Here's how the part is built. I have some questions about the finished solid (model axes, mm). A direction names the side the tool comes from. Round coordinates to 2 decimals unless told otherwise and drop trailing zeros. Put each result on its own line as item: value. Start each with the question number.
1) If I drill on line 1 along X through (y, z) = (80, 9); line 2 along Z through (x, y) = (-166, 528); line 3 along Y through (x, z) = (-142, 5.25), over which ranges is the centre line in solid material (lowest first)? Write a range as [from, to].
2) Which directions (+Z, -Z, +X, -X, +Y, -Y) give clear straight access to the entire face, cutting with the end or side of a thin tool? Please do faces 4 (the cylindrical face through (-140.27, 18.87, 7.1)), 5 (the flat face through (3, 284, 18.4)).
3) Will these pins go through, and if not, where does the flat tip stop? P1, Ø5, axis at y = 528, z = 9.2, coming from the -X side; P2, Ø5.5, axis at y = 560, z = 9.2, coming from the +X side; P3, Ø7, axis at y = 48, z = 9.2, coming from the +X side.
4) We'd pull the mould along Y, two halves only. Please class faces 1 (the conical face through (147.542, 560.536, 18.125)), 2 (the flat face through (3, 0, 9)), 3 (the flat face through (3, 576, 9)): released by +Y, released by -Y, zero draft, split by the parting line, or undercut.
from build123d import *

# Parameters (mm, degrees)
F0_W     = 181
F0_H     = 288
F1_DEPTH = 18.4
F2_D     = 8
F2_DEPTH = 14
F2_TIP   = 2.4034424761
F3_D     = 15
F3_DEPTH = 14
F3_TIP   = 4.5064546427
F5_D     = 7
F5_DEPTH = 28
F5_TIP   = 2.1030121666
F6_D     = 8
F6_DEPTH = 26
F6_TIP   = 2.4034424761


with BuildPart() as f1:
    # F0 (on Top) → F1 (new body)
    with BuildSketch(Plane.XY):
        with Locations((90.5, 144)):
            Rectangle(F0_W, F0_H)
    extrude(amount=F1_DEPTH)

    # F2
    with Locations(Plane(origin=(0, 0, 0), x_dir=(1, 0, 0), z_dir=(0, 0, -1))):
        with Locations((147.2, -80), (147.2, -112)):
            Hole(F2_D / 2, depth=F2_DEPTH)
            with Locations((0, 0, -(F2_DEPTH + F2_TIP / 2))):  # 118° drill point
                Cone(0, F2_D / 2, F2_TIP, mode=Mode.SUBTRACT)

    # F3
    with Locations(Plane(origin=(0, 0, 0), x_dir=(1, 0, 0), z_dir=(0, 0, -1))):
        with Locations((147.2, -16)):
            Hole(F3_D / 2, depth=F3_DEPTH)
            with Locations((0, 0, -(F3_DEPTH + F3_TIP / 2))):  # 118° drill point
                Cone(0, F3_D / 2, F3_TIP, mode=Mode.SUBTRACT)

    # F5
    with Locations(Plane.YZ.offset(181)):
        with Locations((16, 9.2)):
            Hole(F5_D / 2, depth=F5_DEPTH)
            with Locations((0, 0, -(F5_DEPTH + F5_TIP / 2))):  # 118° drill point
                Cone(0, F5_D / 2, F5_TIP, mode=Mode.SUBTRACT)

    # F6
    with Locations(Plane.YZ.offset(181)):
        with Locations((48, 9.2), (208, 9.2)):
            Hole(F6_D / 2, depth=F6_DEPTH)
            with Locations((0, 0, -(F6_DEPTH + F6_TIP / 2))):  # 118° drill point
                Cone(0, F6_D / 2, F6_TIP, mode=Mode.SUBTRACT)

    # F7: F1 across plane


with BuildPart() as f1_1:
    add(f1.part)
    add(f1.part.mirror(Plane.YZ))

    # F8: F1 across face


with BuildPart() as f1_2:
    add(f1_1.part)
    add(f1_1.part.mirror(Plane(origin=(0, 288, 9.2), x_dir=(-1, 0, 0), z_dir=(0, 1, 0))))


solid = f1_2.part
Findings:
1. line 1: x = [-181, -151.2], [-143.2, 143.2], [151.2, 181]
1. line 2: z = [0, 5.2], [13.2, 18.4]
1. line 3: y = [0, 10.6], [21.4, 554.6], [565.4, 576]
2. face 4: -Z
2. face 5: +Z, +X, -X, +Y, -Y
3. P1: stops at x = -154.1
3. P2: stops at x = 140.22
3. P3: stops at x = 154.7
4. face 1: undercut
4. face 2: released by -Y
4. face 3: released by +Y
